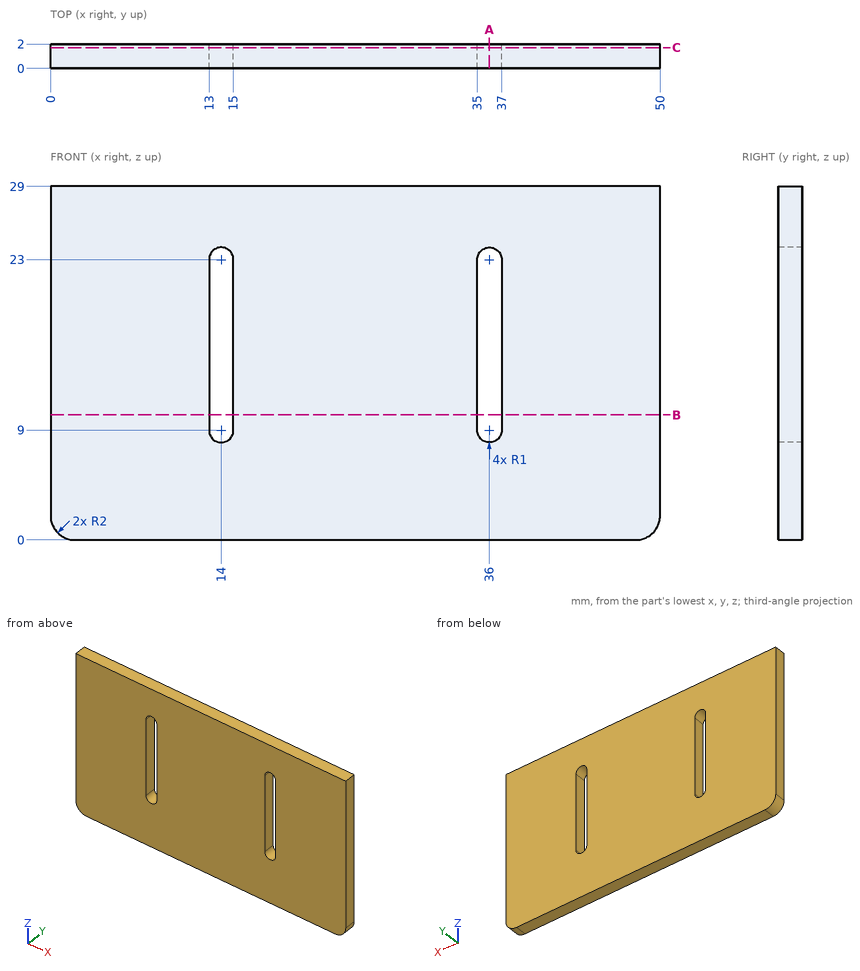
The drawing under review shows one solid part. Ordinate dimensions are in mm from its lowest x, y, z. Give positions to 0.01 mm unless a question says otherwise; leave off trailing zeros. Order: outer loops, then holes, each group sorted by start corner. A loop starts at its lowest first (then second) coordinate and runs counter-clockwise, first axis right, second up. Notation, with made-up numbers: (-16.5, 16) - (9.5, 16) arc R14 ccw to (9.5, 36) - close; hole circle Ø3 at (22, -33.75). An arc over 180 degrees is marked (long way). Answer as a JSON object with one key per item and string values. Group by question number.
Item 1: Take a section at A-A on x = 36. Give the boundary of the cut face in (y, z), and give its area (3 significant figures).
Item 2: Take a section at C-C on y = 1.7. Give the boundary of the cut face in (x, z), and give its area (3 significant figures).
Item 3: Wall thickness on line 1 along X through (y, z) = (0.6, 12.75): over which ranges is the line inside the solid? List them lowest first.
Item 4: Take a section at B-B on z = 10.25. Give the boundary of the cut face in (x, y).
Reported:
{
 "1": {"outline": "(0, 0) - (2, 0) - (2, 8) - (0, 8) - close; (0, 24) - (2, 24) - (2, 29) - (0, 29) - close", "area": "26.0 mm^2"},
 "2": {"outline": "(0, 2) arc R2 ccw to (2, 0) - (48, 0) arc R2 ccw to (50, 2) - (50, 29) - (0, 29) - close; hole (13, 9) arc R1 ccw to (15, 9) - (15, 23) arc R1 ccw to (13, 23) - close; hole (35, 9) arc R1 ccw to (37, 9) - (37, 23) arc R1 ccw to (35, 23) - close", "area": "1,390 mm^2"},
 "3": {"line 1": "0 to 13, 15 to 35, 37 to 50"},
 "4": {"outline": "(0, 0) - (13, 0) - (13, 2) - (0, 2) - close; (15, 0) - (35, 0) - (35, 2) - (15, 2) - close; (37, 0) - (50, 0) - (50, 2) - (37, 2) - close"}
}
